```python
from build123d import *

# Parameters (mm, degrees)
PAD003_DEPTH         = 5.5
POCKET004_DEPTH      = 2.951
POCKET004_DEPTH_BACK = 2.951
SKETCH013_R          = 0.8
PAD006_DEPTH         = 0.7
FILLET_R             = 0.5
CHAMFER004_SIZE      = 0.6


with BuildPart() as part:
    # Sketch004 → Pad003 (new body)
    with BuildSketch(Plane.XY):
        with BuildLine():
            ThreePointArc((2.2, -1.9653244007), (0, 2.95), (-2.2, -1.9653244007))
            Line((-2.2, -1.9653244007), (2.2, -1.9653244007))
        make_face()
    extrude(amount=PAD003_DEPTH)

    # Sketch014 → Pocket004 (cut, two sides)
    with BuildSketch(Plane.YZ) as pocket004_sk:
        Polygon((-1.97, 5.5), (-1.67, 4.5), (-1.67, 2.8), (-1.22, 1.8), (4, 1.8), (4, 5.5), align=None)
    extrude(amount=-POCKET004_DEPTH, mode=Mode.SUBTRACT)
    extrude(pocket004_sk.sketch, amount=POCKET004_DEPTH_BACK, mode=Mode.SUBTRACT)

    # Sketch013 (on Face7 of Pocket004) → Pad006 (join)
    with BuildSketch(Plane.XY.offset(1.8)):
        with Locations((0, 0.5)):
            Circle(SKETCH013_R)
    extrude(amount=PAD006_DEPTH)

    # Fillet
    fillet_edges = [part.edges().sort_by_distance(p)[0] for p in [
        (-0.8, 0.5, 2.5),
    ]]
    fillet(fillet_edges, radius=FILLET_R)

    # Chamfer004
    chamfer004_edges = [part.edges().sort_by_distance(p)[0] for p in [
        (0, 2.95, 0),
        (0, -1.965324, 0),
    ]]
    chamfer(chamfer004_edges, length=CHAMFER004_SIZE)


with BuildPart() as part_1:
    # Body024 placement: moved
    add(part.part.moved(Location((0, 30, 0))))


solid = part_1.part
```
The listing builds one solid part. Answer for the finished solid, in the listing's coordinates (mm). A direction names the side the tool comes from. Coordinates: 2 decimals unless noted, no trailing zeros. Loops run counter-clockwise (first coordinate to the right, second up) from the corner with the lowest first, then second, coordinate; pieces in that order, holes last. Notation, with made-up numbers: (54.5, 8.25) - (105.5, 8.25) arc R8 ccw to (105.5, 13.25) - close; hole circle Ø9 at (-17, 1.25). An arc over 180 degrees is marked (long way). Use a Markdown table: item, result. Add a question column.
1) The mould has two halves that part along Y. Classify faces 4 (the flat face through (0.04, 28.55, 2.31)), 5 (the flat face through (0.034, 28.213, 4.89)), 6 (the conical face through (0.08, 32.51, 0.16)): released by +Y, released by -Y, zero draft, split by the parting line, or undercut.
2) Given pin 1 (1.4 mm diameter, centred on x = -0.5, z = 4, fed in from +Y); pin 2 (2 mm diameter, centred on x = 0, y = 32, fed in from +Z), each flat-ended and moving along its own axis, determine where each tip first touches the part or whether it passes through.
3) Find the intervals of material crossed by line 1 (Z direction, x = -0.8, y = 30.8); line 2 (Y direction, x = -0.85, z = 3.35); line 3 (Y direction, x = 1.7, z = 2.35), in increasing order.
4) The part is cut by section B-B, the plane z = 0.4. Give the vertices of the cut face in (x, y).
5) The part is cut by section A-A, the plane z = 4.9. Give the vertices of the cut face in (x, y).
6) For faces 1 (the flat face through (0, 28.33, 4)), 2 (the flat face through (-1, 30, 1.8)), 3 (the cylindrical face through (0.53, 32.9, 1.4)), determine the directions among +Z, -Z, +X, -X, +Y, -Y from which every point of the face is accessible in a straight line to the end or side of a thin tool.
Here are the results:
| question | item | result |
|---|---|---|
| 1 | face 4 | undercut |
| 1 | face 5 | released by +Y |
| 1 | face 6 | split by the parting line |
| 2 | pin 1 | stops at y = 28.33 |
| 2 | pin 2 | stops at z = 2.46 |
| 3 | line 1 | z = 0 to 1.8 |
| 3 | line 2 | y = 28.03 to 28.33 |
| 3 | line 3 | y = 28.03 to 28.53 |
| 4 | outline | (-2.11, 28.23) - (2.11, 28.23) arc R2.75 ccw (long way) to start |
| 5 | outline | (-2.34, 28.21) arc R2.95 ccw to (-2.2, 28.03) - (2.2, 28.03) arc R2.95 ccw to (2.34, 28.21) - close |
| 6 | face 1 | +Z, +X, -X, +Y |
| 6 | face 2 | +Z |
| 6 | face 3 | +Z, -Z |
